```python
from build123d import *

# Parameters (mm, degrees)
BOSS_EXTRUDE1_DEPTH = 35
SKETCH3_W           = 11.2
SKETCH3_H           = 6
CUT_EXTRUDE1_DEPTH  = 58.584830686
SKETCH4_R           = 3.05
CUT_EXTRUDE2_DEPTH  = 61.713451947
FILLET1_R           = 2.5
FILLET4_R           = 1


# Some blends are built 0.0001 mm under size
with BuildPart() as part:
    # Sketch2 → Boss-Extrude1 (new, symmetric)
    with BuildSketch(Plane.XY):
        Polygon((0, 0), (30, 34.511052217), (30, -9), (-25, -9), (-25, -5), (0, -5), align=None)
    extrude(amount=BOSS_EXTRUDE1_DEPTH, both=True)

    # Sketch3 → Cut-Extrude1 (cut, through all)
    with BuildSketch(Plane(origin=(0, 0, 0), x_dir=(0, 0, -1), z_dir=(1, 0, 0))):
        with Locations((0, -6)):
            Rectangle(SKETCH3_W, SKETCH3_H)
    extrude(amount=-CUT_EXTRUDE1_DEPTH, mode=Mode.SUBTRACT)

    # Sketch4 → Cut-Extrude2 (cut, through all)
    with BuildSketch(Plane(origin=(0, -5, 0), x_dir=(1, 0, 0), z_dir=(0, 1, 0))):
        with Locations(Location((-15, -20, 0), (0, 0, 270))):
            Circle(SKETCH4_R)
        with Locations(Location((-15, 20, 0), (0, 0, 90))):
            Circle(SKETCH4_R)
    extrude(amount=-CUT_EXTRUDE2_DEPTH, mode=Mode.SUBTRACT)

    # Fillet1
    # the kernel refuses this fillet: 2.5 mm, written as the material it adds along each edge
    with BuildSketch(Plane(origin=(0, -5, -35), x_dir=(0, 1, 0), z_dir=(0, 0, 1)), Plane(origin=(0, -5, 5.6), x_dir=(0, 1, 0), z_dir=(0, 0, 1))) as fillet1_piece_1:
        with BuildLine():
            CenterArc((FILLET1_R, FILLET1_R), FILLET1_R, 180, 90)
            Line((0, FILLET1_R), (0, 0))
            Line((0, 0), (FILLET1_R, 0))
        make_face()
    extrude(amount=29.4)
    # the kernel refuses this fillet: 2.5 mm, written as the material it takes off along each edge
    with BuildSketch(Plane(origin=(27.5, -6.5, 32.5), x_dir=(1, 0, 0), z_dir=(0, 0, 1))) as fillet1_2_piece_1_section:
        Polygon((0, 0), (FILLET1_R, 0), (FILLET1_R, -FILLET1_R), (0, -FILLET1_R), align=None)
    fillet1_2_piece_1 = extrude(amount=FILLET1_R, mode=Mode.PRIVATE)
    fillet1_2_piece_1 = fillet1_2_piece_1 - Plane(origin=(27.5, -6.5, 32.5), x_dir=(-0.7071067811865476, 0.7071067811865474, 0), z_dir=(0, 0, 1)) * Sphere(FILLET1_R, mode=Mode.PRIVATE)
    add(fillet1_2_piece_1, mode=Mode.SUBTRACT)
    with BuildSketch(Plane(origin=(27.5, -6.5, -32.5), x_dir=(0, 0, -1), z_dir=(1, 0, 0))) as fillet1_2_piece_2_section:
        Polygon((0, 0), (FILLET1_R, 0), (FILLET1_R, -FILLET1_R), (0, -FILLET1_R), align=None)
    fillet1_2_piece_2 = extrude(amount=FILLET1_R, mode=Mode.PRIVATE)
    fillet1_2_piece_2 = fillet1_2_piece_2 - Plane(origin=(27.5, -6.5, -32.5), x_dir=(0, 0.7071067811865475, 0.7071067811865475), z_dir=(1, 0, 0)) * Sphere(FILLET1_R, mode=Mode.PRIVATE)
    add(fillet1_2_piece_2, mode=Mode.SUBTRACT)
    with BuildSketch(Plane(origin=(30, -9, 32.5), x_dir=(-1, 0, 0), z_dir=(0, 0, -1))) as fillet1_2_piece_3:
        with BuildLine():
            CenterArc((FILLET1_R, FILLET1_R), FILLET1_R, 180, 90)
            Line((0, FILLET1_R), (0, 0))
            Line((0, 0), (FILLET1_R, 0))
        make_face()
    extrude(amount=65, mode=Mode.SUBTRACT)
    with BuildSketch(Plane(origin=(30, 40.761052217, -35), x_dir=(0, 0, 1), z_dir=(0, -1, 0)), Plane(origin=(30, 40.761052217, 35), x_dir=(-1, 0, 0), z_dir=(0, -1, 0))) as fillet1_2_piece_4:
        with BuildLine():
            CenterArc((FILLET1_R, FILLET1_R), FILLET1_R, 180, 90)
            Line((0, FILLET1_R), (0, 0))
            Line((0, 0), (FILLET1_R, 0))
        make_face()
    extrude(amount=47.261052217, mode=Mode.SUBTRACT)
    with BuildSketch(Plane(origin=(27.5, -9, 35), x_dir=(0, 1, 0), z_dir=(-1, 0, 0)), Plane(origin=(27.5, -9, -35), x_dir=(0, 0, 1), z_dir=(-1, 0, 0))) as fillet1_2_piece_5:
        with BuildLine():
            CenterArc((FILLET1_R, FILLET1_R), FILLET1_R, 180, 90)
            Line((0, FILLET1_R), (0, 0))
            Line((0, 0), (FILLET1_R, 0))
        make_face()
    extrude(amount=58.75, mode=Mode.SUBTRACT)
    # the kernel refuses this fillet: 2.5 mm, written as the material it takes off along each edge
    with BuildSketch(Plane(origin=(0, -2.5, 35), x_dir=(0, 0, -1), z_dir=(0, 1, 0))) as fillet1_3_piece_1:
        with BuildLine():
            CenterArc((FILLET1_R, -FILLET1_R), FILLET1_R, 90, 90)
            Line((0, -FILLET1_R), (0, 0))
            Line((0, 0), (FILLET1_R, 0))
        make_face()
    extrude(amount=8.75, mode=Mode.SUBTRACT)
    with BuildSketch(Plane(origin=(0, -2.5, -35), x_dir=(0, 0, 1), z_dir=(0, 1, 0))) as fillet1_3_piece_2:
        with BuildLine():
            CenterArc((FILLET1_R, FILLET1_R), FILLET1_R, 180, 90)
            Line((0, FILLET1_R), (0, 0))
            Line((0, 0), (FILLET1_R, 0))
        make_face()
    extrude(amount=8.75, mode=Mode.SUBTRACT)
    with BuildSketch(Plane(origin=(-31.25, -5, 35), x_dir=(0, -1, 0), z_dir=(1, 0, 0))) as fillet1_3_piece_3:
        with BuildLine():
            CenterArc((FILLET1_R, FILLET1_R), FILLET1_R, 180, 90)
            Line((0, FILLET1_R), (0, 0))
            Line((0, 0), (FILLET1_R, 0))
        make_face()
    extrude(amount=28.75, mode=Mode.SUBTRACT)
    with BuildSketch(Plane(origin=(-31.25, -5, -35), x_dir=(0, -1, 0), z_dir=(1, 0, 0))) as fillet1_3_piece_4:
        with BuildLine():
            CenterArc((FILLET1_R, -FILLET1_R), FILLET1_R, 90, 90)
            Line((0, -FILLET1_R), (0, 0))
            Line((0, 0), (FILLET1_R, 0))
        make_face()
    extrude(amount=28.75, mode=Mode.SUBTRACT)
    with BuildSketch(Plane(origin=(-2.5, -2.5, -35), x_dir=(1, 0, 0), z_dir=(0, 1, 0))) as fillet1_3_piece_5:
        with BuildLine():
            CenterArc((2.5 + FILLET1_R, -FILLET1_R), FILLET1_R, 90, 90)
            Line((2.5, -FILLET1_R), (2.5, 0))
            Line((2.5, 0), (2.5 + FILLET1_R, 0))
        make_face()
    revolve(axis=Axis((-2.5, -2.5, -35), (0, 0, -1)), revolution_arc=90, mode=Mode.SUBTRACT)
    with BuildSketch(Plane(origin=(-2.5, -2.5, 35), x_dir=(1, 0, 0), z_dir=(0, 1, 0))) as fillet1_3_piece_6:
        with BuildLine():
            CenterArc((2.5 + FILLET1_R, FILLET1_R), FILLET1_R, 180, 90)
            Line((2.5, FILLET1_R), (2.5, 0))
            Line((2.5, 0), (2.5 + FILLET1_R, 0))
        make_face()
    revolve(axis=Axis((-2.5, -2.5, 35), (0, 0, -1)), revolution_arc=90, mode=Mode.SUBTRACT)

    # Fillet4
    fillet4_edges = [part.edges().sort_by_distance(p)[0] for p in [
        (-25, -8.436491673, -34.08113883),
        (-25, -8.436491673, 34.08113883),
        (-25, -9, -19.05),
        (-25, -9, 19.05),
    ]]
    fillet(fillet4_edges, radius=FILLET4_R - 0.0001)  # a hair under: the kernel refuses the full size


solid = part.part
```
Check sheet for the modelled part. Datum: model origin and axes. Units: mm. A direction names the side the tool comes from. Coordinates: 2 decimals unless noted, no trailing zeros. Loops run counter-clockwise (first coordinate to the right, second up) from the corner with the lowest first, then second, coordinate; pieces in that order, holes last.
1) Gauge pin test, flat ends, axial feed: pin 1 (4 mm diameter, centred on x = 0, z = 9, fed in from +Y); pin 2 (12 mm diameter, centred on x = -8, z = 7, fed in from +Y); pin 3 (18 mm diameter, centred on x = -10.5, z = -15.5, fed in from +Y). Record the tip position at first contact, or that the pin passes through.
2) Release check for a two-part mould opening along Z. For faces 1 (the face through (-11, -5, 19)), 2 (the face through (17, 9, -35)), 3 (the face through (-13, -7, -5.6)) record: released by +Z, released by -Z, zero draft, split by the parting line, or undercut.
3) Access from +Z, -Z, +X, -X, +Y, -Y to the whole of each face (thin tool, end or side, straight path). Record for faces 4 (the face through (0, -3, 0)), 5 (the face through (-11, -5, -19)), 6 (the face through (-13.91, -5.58, -34.1)), 7 (the face through (29.287, 14.293, 34.248)), 8 (the face through (1, -0.4, 34.5)).
4) Sectioned sample at C-C (z = -12.5). Record the boundary of the cut face in (x, y), and give its area (3 significant figures).
5) Material ranges on probe 1 along Z at (x, y) = (-5, -7); probe 2 along Y at (x, z) = (-13, -28.5); probe 3 along X at (y, z) = (26.5, -10), recorded low to high.
6) Sectioned sample at D-D (y = 24). Record the boundary of the cut face in (x, z), and give its area (3 significant figures).
7) Sectioned sample at B-B (z = 20). Record the boundary of the cut face in (x, y), and give its area (3 significant figures).
8) Sectioned sample at A-A (x = -15). Record the boundary of the cut face in (y, z), and give its area (3 significant figures).
Check sheet entries:
1. pin 1: stops at y = 2.3
1. pin 2: stops at y = -4.95
1. pin 3: stops at y = -4.79
2. face 1: zero draft
2. face 2: released by -Z
2. face 3: undercut
3. face 4: -X, +Y
3. face 5: +Z, -Z, -X, +Y
3. face 6: -Z, -X, +Y
3. face 7: +Z, +X, +Y, -Y
3. face 8: +Z, -X, +Y
4. outline: (-25, -8) arc R1 ccw to (-24, -9) - (27.5, -9) arc R2.5 ccw to (30, -6.5) - (30, 34.51) - (0, 0) - (0, -2.5) arc R2.5 cw to (-2.5, -5) - (-25, -5) - close
4. area: 887 mm2
5. probe 1: z = -34.95 to -5.6, 5.6 to 34.95
5. probe 2: y = -9 to -5
5. probe 3: x = 23.04 to 30
6. outline: (20.86, -35) - (27.5, -35) arc R2.5 ccw to (30, -32.5) - (30, 32.5) arc R2.5 ccw to (27.5, 35) - (20.86, 35) - close
6. area: 637 mm2
7. outline: (-25, -8) arc R1 ccw to (-24, -9) - (-18.05, -9) - (-18.05, -5) - (-25, -5) - close; (-11.95, -9) - (27.5, -9) arc R2.5 ccw to (30, -6.5) - (30, 34.51) - (0, 0) - (0, -2.5) arc R2.5 cw to (-2.5, -5) - (-11.95, -5) - close
7. area: 863 mm2
8. outline: (-9, -32.5) arc R2.5 ccw to (-7, -34.95) arc R2.5 ccw to (-5, -32.5) - (-5, -23.05) - (-9, -23.05) - close; (-9, -16.95) - (-5, -16.95) - (-5, -5.6) - (-9, -5.6) - close; (-9, 5.6) - (-5, 5.6) - (-5, 16.95) - (-9, 16.95) - close; (-9, 23.05) - (-5, 23.05) - (-5, 32.5) arc R2.5 ccw to (-7, 34.95) arc R2.5 ccw to (-9, 32.5) - close
8. area: 181 mm2
